```python
from build123d import *

# Parameters (mm, degrees)
BOSS_EXTRUDE1_DEPTH = 6
SKETCH4_R           = 1.25
CUT_EXTRUDE1_DEPTH  = 6


with BuildPart() as part:
    # Sketch1 → Boss-Extrude1 (new body)
    with BuildSketch(Plane(origin=(0, 0, 0), x_dir=(0, 0, -1), z_dir=(1, 0, 0))):
        with BuildLine():
            Line((41.203205101, 15.688911622), (43.203205101, 17.688911622))
            Line((43.203205101, 17.688911622), (65.948748697, 17.688911622))
            Line((65.948748697, 17.688911622), (65.948748697, -32.311088378))
            Line((65.948748697, -32.311088378), (43.203205101, -32.311088378))
            Line((43.203205101, -32.311088378), (41.203205101, -30.311088378))
            Line((41.203205101, -30.311088378), (41.203205101, -23.561088378))
            Line((41.203205101, -23.561088378), (43.880106331, -23.561088378))
            Line((43.880106331, -23.561088378), (44.81485523, -24.633587377))
            Line((44.81485523, -24.633587377), (44.81485523, -27.311088378))
            Line((44.81485523, -27.311088378), (56.547992273, -27.311088378))
            Line((56.547992273, -27.311088378), (56.547992273, -25.708962028))
            ThreePointArc((56.547992273, -25.708962028), (62.834374894, -16.931491254), (57.934329164, -7.311088378))
            ThreePointArc((57.934329164, -7.311088378), (62.834374894, 2.309314498), (56.547992273, 11.086785272))
            Line((56.547992273, 11.086785272), (56.547992273, 12.688911622))
            Line((56.547992273, 12.688911622), (44.81485523, 12.688911622))
            Line((44.81485523, 12.688911622), (44.81485523, 10.011410621))
            Line((44.81485523, 10.011410621), (43.880106331, 8.938911622))
            Line((43.880106331, 8.938911622), (41.203205101, 8.938911622))
            Line((41.203205101, 8.938911622), (41.203205101, 15.688911622))
        make_face()
    extrude(amount=BOSS_EXTRUDE1_DEPTH)

    # Sketch4 → Cut-Extrude1 (cut)
    with BuildSketch(Plane(origin=(0, 0, -65.948748697), x_dir=(-1, 0, 0), z_dir=(0, 0, -1))):
        with Locations((-3, 15.188911622)):
            Circle(SKETCH4_R)
        with Locations(Location((-3, -29.622535768, 0), (0, 0, 180))):
            Circle(SKETCH4_R)
    extrude(amount=-CUT_EXTRUDE1_DEPTH, mode=Mode.SUBTRACT)


solid = part.part
```
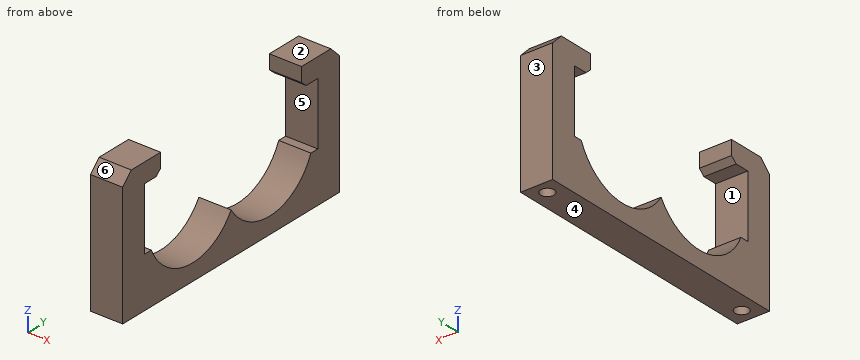
Work out the finished part from the listing and answer in its coordinate system (mm). Face numbers are marked on the shaded views. A direction names the side the tool comes from. Give positions to 0.01 mm unless a question says otherwise; leave off trailing zeros. Loops run counter-clockwise (first coordinate to the right, second up) from the corner with the lowest first, then second, coordinate; pieces in that order, holes last. Notation, with made-up numbers: (82.25, 9) -> (121.25, 9) arc R13 ccw to (121.25, 26) -> close; hole circle Ø3 at (23.5, -6). An arc over 180 degrees is marked (long way). Use CSV: the item, a comma, the result in double quotes.
1. The part is cut by section D-D (y = 6). Write down the section's boundary in (x, z), then the cut area to 3 significant figures.
Found:
outline,"(0, -65.95) -> (6, -65.95) -> (6, -61.85) -> (0, -61.85) -> close"
area,"24.6 mm^2"
2. The part is cut by section C-C (y = -11). Write down the section's boundary in (x, z).
Found:
outline,"(0, -65.95) -> (6, -65.95) -> (6, -61.5) -> (0, -61.5) -> close"
3. The part is cut by section A-A (z = -42.75). Write down the section's boundary in (x, y).
Found:
outline,"(0, -31.86) -> (6, -31.86) -> (6, -23.56) -> (0, -23.56) -> close; (0, 8.94) -> (6, 8.94) -> (6, 17.24) -> (0, 17.24) -> close"
4. The mould has two halves that part along Z. Classify the marked faces 1, 2, 3 and 4: +Z half, -Z half, draft (parallel to the pull), parting line (faces both ways), or undercut.
Found:
face 1,"undercut"
face 2,"+Z half"
face 3,"draft"
face 4,"-Z half"
5. Straight lines are drawn through the part: line 1 (Y direction, x = 1.9, z = -55.25); line 2 (Y direction, x = 1.7, z = -60); line 3 (Y direction, x = 3, z = -63.55). For each, find the intervals that lie inside material, in ascending order.
Found:
line 1,"-32.31 to -27.31, 12.69 to 17.69"
line 2,"-32.31 to -23.31, -8.99 to -5.63, 8.69 to 17.69"
line 3,"-32.31 to -30.87, -28.37 to 13.94, 16.44 to 17.69"
6. The part is cut by section B-B (x = 3). Write down the section's boundary in (y, z), then the cut area to 3 significant figures.
Found:
outline,"(-32.31, -65.95) -> (-30.87, -65.95) -> (-30.87, -59.95) -> (-28.37, -59.95) -> (-28.37, -65.95) -> (13.94, -65.95) -> (13.94, -59.95) -> (16.44, -59.95) -> (16.44, -65.95) -> (17.69, -65.95) -> (17.69, -43.2) -> (15.69, -41.2) -> (8.94, -41.2) -> (8.94, -43.88) -> (10.01, -44.81) -> (12.69, -44.81) -> (12.69, -56.55) -> (11.09, -56.55) arc R10.39 cw to (-7.31, -57.93) arc R10.39 cw to (-25.71, -56.55) -> (-27.31, -56.55) -> (-27.31, -44.81) -> (-24.63, -44.81) -> (-23.56, -43.88) -> (-23.56, -41.2) -> (-30.31, -41.2) -> (-32.31, -43.2) -> close"
area,"442 mm^2"
7. Flat-ended cylindrical pins translate along their axes: pin 1 Ø1.3 at (x, z) = (4, -42) entering from +Y; pin 2 Ø0.8 at (x, z) = (3.5, -42.5) entering from -Y. Find the tip coordinate at first contact, or state that the pin passes through.
Found:
pin 1,"y = 17.14"
pin 2,"y = -32.01"
8. A tool of negligible diameter and unlimited length cuts with its end or side. For the marked faces 5 and 6, from which of +Z, -Z, +X, -X, +Y, -Y can it reach the whole face along a straight path? Write none if from no direction.
Found:
face 5,"+X, -X"
face 6,"+Z, +X, -X, -Y"
